```python
from build123d import *

# Parameters (mm, degrees)
SKETCH1_W           = 19.5
SKETCH1_H           = 13.556349186
SKETCH1_R           = 1.75
BOSS_EXTRUDE1_DEPTH = 5
SKETCH2_W           = 6
SKETCH2_H           = 3
BOSS_EXTRUDE2_DEPTH = 2
SKETCH3_W           = 6
SKETCH3_H           = 13.556349186
SKETCH3_R           = 1
BOSS_EXTRUDE3_DEPTH = 5
CHAMFER1_SIZE       = 4
CHAMFER2_SIZE       = 6


with BuildPart() as part:
    # Sketch1 → Boss-Extrude1 (new body)
    with BuildSketch(Plane.XY):
        with Locations((-25.671858451, -15.778174593)):
            Rectangle(SKETCH1_W, SKETCH1_H)
        with Locations((-20.921858451, -15.778174593)):
            Circle(SKETCH1_R, mode=Mode.SUBTRACT)
    extrude(amount=BOSS_EXTRUDE1_DEPTH)

    # Sketch2 → Boss-Extrude2 (add)
    with BuildSketch(Plane(origin=(0, 0, 0), x_dir=(-1, 0, 0), z_dir=(0, 0, -1))):
        with Locations((32.421858451, -15.778174593)):
            Rectangle(SKETCH2_W, SKETCH2_H)
    extrude(amount=BOSS_EXTRUDE2_DEPTH)

    # Sketch3 → Boss-Extrude3 (add)
    with BuildSketch(Plane.ZY.offset(35.421858451)):
        with Locations((8, -15.778174593)):
            Rectangle(SKETCH3_W, SKETCH3_H)
        with Locations((8, -15.778174593)):
            Circle(SKETCH3_R, mode=Mode.SUBTRACT)
    extrude(amount=-BOSS_EXTRUDE3_DEPTH)

    # Chamfer1
    chamfer1_edges = [part.edges().sort_by_distance(p)[0] for p in [
        (-32.921858451, -9, 11),
        (-32.921858451, -22.556349186, 11),
    ]]
    chamfer(chamfer1_edges, length=CHAMFER1_SIZE)

    # Chamfer2
    # the kernel refuses this chamfer: 6 mm, written as the material it adds along each edge
    with BuildSketch(Plane(origin=(-30.421858451, -22.556349186, 5), x_dir=(-0.0274958766105862, 0, 0.9996219169112968), z_dir=(0, 1, 0))) as chamfer2_piece_1_section:
        Polygon((CHAMFER2_SIZE * 0.999621916911, CHAMFER2_SIZE * 0.0274958766106), (-CHAMFER2_SIZE * 0.0274958766106, CHAMFER2_SIZE * 0.999621916911), (0, 0), align=None)
    chamfer2_piece_1 = extrude(amount=13.556349186, mode=Mode.PRIVATE)
    chamfer2_piece_1 = split(chamfer2_piece_1, bisect_by=Plane(origin=(-28.301106776, -12.243149914, 10.243149914), z_dir=(0, -0.7071067811865477, -0.7071067811865474)), keep=Keep.TOP, mode=Mode.PRIVATE)
    chamfer2_piece_1 = split(chamfer2_piece_1, bisect_by=Plane(origin=(-28.301106776, -15.778174309, 11), z_dir=(0, 0, -1)), keep=Keep.TOP, mode=Mode.PRIVATE)
    chamfer2_piece_1 = split(chamfer2_piece_1, bisect_by=Plane(origin=(-28.301106776, -19.313198988, 10.243150199), z_dir=(0, 0.7071067811865474, -0.7071067811865477)), keep=Keep.TOP, mode=Mode.PRIVATE)
    chamfer2_piece_1 = chamfer2_piece_1 - Plane(origin=(-28.301106776, -15.778174593, 8), x_dir=(0, 0, 1), z_dir=(-1, 0, 0)) * Cylinder(1, 52, mode=Mode.PRIVATE)
    add(chamfer2_piece_1)


solid = part.part
```
Part model, mm, in its own coordinate system. A direction names the side the tool comes from. Round coordinates to 2 decimals unless told otherwise and drop trailing zeros. Loops run counter-clockwise (first coordinate to the right, second up) from the corner with the lowest first, then second, coordinate; pieces in that order, holes last. Notation, with made-up numbers: (53, -39) -> (64, -39) arc R18 cw to (64, -9) -> close; hole circle Ø2 at (-18.75, 82.5). An arc over 180 degrees is marked (long way). Use one line per item in the form item = value. Start each with the question number.
Item 1: Band-saw the part on C-C (z = 8). List the corners of the cut face in (x, y).
Item 2: Band-saw the part on B-B (x = -21). List the corners of the cut face in (y, z).
Item 3: Band-saw the part on D-D (x = -28). List the corners of the cut face in (y, z), plus the area to 3 significant figures.
Item 4: Drill centre lines: line 1 along X through (y, z) = (-10.5, 7); line 2 along Y through (x, z) = (-20, 1); line 3 along Y through (x, z) = (-28.5, 7.5). Where is each one in solid material? Low to high.
Item 5: Two-plate mould, pull along Y, no slides. Class faces 1 (the flat face through (-26, -9, 3)), 2 (the flat face through (-35.422, -16, 4)), 3 (the cylindrical face through (-30.94, -15.73, 7)): released by +Y, released by -Y, zero draft, split by the parting line, or undercut.
Item 6: Tool access for faces 4 (the flat face through (-19, -17, 5)), 5 (the flat face through (-32, -14.278, -1)), 6 (the flat face through (-29.422, -16, -1)), 7 (the flat face through (-32, -17.278, -1)): list every direction of +Z, -Z, +X, -X, +Y, -Y with a clear straight run to the whole face (end or side of a thin tool).
Item 7: Band-saw the part on A-A (y = -14.5). List the corners of the cut face in (x, z).
Item 8: Drop flat-ended pins along their axis: pin 1 Ø6 at (x, y) = (-20.5, -13) entering from -Z; pin 2 Ø4.5 at (x, y) = (-20.92, -15.78) entering from +Z; pin 3 Ø6 at (x, y) = (-23, -11.5) entering from +Z. Give the stop position or say it passes through.
Data:
q1.outline = (-35.42, -21.56) -> (-27.42, -21.56) -> (-27.42, -16.78) -> (-35.42, -16.78) -> close; (-35.42, -14.78) -> (-27.42, -14.78) -> (-27.42, -10) -> (-35.42, -10) -> close
q2.outline = (-22.56, 0) -> (-17.53, 0) -> (-17.53, 5) -> (-22.56, 5) -> close; (-14.03, 0) -> (-9, 0) -> (-9, 5) -> (-14.03, 5) -> close
q3.outline = (-22.56, 0) -> (-9, 0) -> (-9, 7) -> (-10.58, 8.58) -> (-14.96, 8.58) arc R1 cw (long way) to (-16.59, 8.58) -> (-20.98, 8.58) -> (-22.56, 7) -> close
q3.area = 111 mm^2
q4.line_1 = -35.42 to -26.42
q4.line_2 = -22.56 to -17.27, -14.29 to -9
q4.line_3 = -22.06 to -16.64, -14.91 to -9.5
q5.face_1 = released by +Y
q5.face_2 = zero draft
q5.face_3 = undercut
q6.face_4 = +Z, +X, +Y, -Y
q6.face_5 = -Z, +X, -X, +Y
q6.face_6 = -Z, +X, +Y, -Y
q6.face_7 = -Z, +X, -X, -Y
q7.outline = (-35.42, -2) -> (-29.42, -2) -> (-29.42, 0) -> (-22.12, 0) -> (-22.12, 5) -> (-24.42, 5) -> (-30.42, 11) -> (-35.42, 11) -> close; (-19.73, 0) -> (-15.92, 0) -> (-15.92, 5) -> (-19.73, 5) -> close
q8.pin_1 = 0
q8.pin_2 = 5
q8.pin_3 = 6.58
